from build123d import *

# Parameters (mm, degrees)
SKETCH1_W                      = 50.8
SKETCH1_H                      = 19.05
BOSS_EXTRUDE1_DEPTH            = 25.4
CUT_EXTRUDE1_DEPTH             = 38.162422217
CUT_EXTRUDE1_DEPTH_BACK        = 38.1
M4X0_7_TAPPED_HOLE1_D          = 3.3
M4X0_7_TAPPED_HOLE1_DEPTH      = 10.1092
M4X0_7_TAPPED_HOLE1_TIP        = 0.991420021
BOSS_EXTRUDE4_DEPTH            = 12.7
M2X0_4_TAPPED_HOLE1_AT_2_COUNT = 2
M2X0_4_TAPPED_HOLE1_AT_2_PITCH = 12.7
CUT_EXTRUDE2_DEPTH             = 12.7


with BuildPart() as part:
    # Sketch1 → Boss-Extrude1 (new body)
    with BuildSketch(Plane.XY):
        Rectangle(SKETCH1_W, SKETCH1_H)
    extrude(amount=BOSS_EXTRUDE1_DEPTH)

    # Sketch2 → Cut-Extrude1 (cut, two sides)
    with BuildSketch(Plane(origin=(0, 0, 0), x_dir=(-1, 0, 0), z_dir=(0, 0, -1))) as cut_extrude1_sk:
        Polygon((-6.461803399, -9.525), (-6.35, -9.525), (-12.7, 3.175), (12.7, 3.175), (6.35, -9.525), (6.461803399, -9.525), (12.861803399, 3.275), (-12.861803399, 3.275), align=None)
        Polygon((-12.7, 3.175), (-6.35, -9.525), (6.35, -9.525), (12.7, 3.175), align=None)
    extrude(amount=CUT_EXTRUDE1_DEPTH, mode=Mode.SUBTRACT)
    extrude(cut_extrude1_sk.sketch, amount=-CUT_EXTRUDE1_DEPTH_BACK, mode=Mode.SUBTRACT)

    # M4x0.7 Tapped Hole1
    with Locations(Plane(origin=(0, 9.525, 0), x_dir=(1, 0, 0), z_dir=(0, 1, 0))):
        with Locations((-19.05, -12.7), (19.05, -12.7)):
            Hole(M4X0_7_TAPPED_HOLE1_D / 2, depth=M4X0_7_TAPPED_HOLE1_DEPTH)
            with Locations((0, 0, -(M4X0_7_TAPPED_HOLE1_DEPTH + M4X0_7_TAPPED_HOLE1_TIP / 2))):  # 118° drill point
                Cone(0, M4X0_7_TAPPED_HOLE1_D / 2, M4X0_7_TAPPED_HOLE1_TIP, mode=Mode.SUBTRACT)

    # Sketch8 → Boss-Extrude4 (add)
    with BuildSketch(Plane.XZ.offset(9.525)):
        Polygon((25.4, 25.4), (63.5, -6.35), (63.5, -31.75), (25.4, 0), align=None)
    boss_extrude4 = extrude(amount=-BOSS_EXTRUDE4_DEPTH)

    # Sketch19 → M2x0.4 Tapped Hole1 (revolve, cut)
    with BuildSketch(Plane(origin=(63.5, -3.175, -22.225), x_dir=(0, 0, -1), z_dir=(0, 1, 0))):
        Polygon((0, 0), (0, 6.830688495), (0.8, 6.35), (0.8, 0), align=None)
    m2x0_4_tapped_hole1 = revolve(axis=Axis((69.85, -3.175, -22.225), (-1, 0, 0)), mode=Mode.SUBTRACT)

    # M2x0.4 Tapped Hole1 at 2: M2x0.4 Tapped Hole1 ×2
    with Locations(*[(0, 0, i * M2X0_4_TAPPED_HOLE1_AT_2_PITCH) for i in range(1, M2X0_4_TAPPED_HOLE1_AT_2_COUNT)]):
        add(m2x0_4_tapped_hole1, mode=Mode.SUBTRACT)

    # Sketch20 → Cut-Extrude2 (cut)
    with BuildSketch(Plane(origin=(0, 3.175, 0), x_dir=(1, 0, 0), z_dir=(0, 1, 0))):
        Polygon((57.404, 26.67), (63.5, 26.67), (63.5, 31.75), align=None)
    cut_extrude2 = extrude(amount=-CUT_EXTRUDE2_DEPTH, mode=Mode.SUBTRACT)

    # Mirror1: Boss-Extrude4, M2x0.4 Tapped Hole1, Cut-Extrude2 across plane
    add(boss_extrude4.mirror(Plane(origin=(0, 0, 0), x_dir=(0, 0, 1), z_dir=(1, 0, 0))))
    add(m2x0_4_tapped_hole1.mirror(Plane(origin=(0, 0, 0), x_dir=(0, 0, 1), z_dir=(1, 0, 0))), mode=Mode.SUBTRACT)
    add(cut_extrude2.mirror(Plane(origin=(0, 0, 0), x_dir=(0, 0, 1), z_dir=(1, 0, 0))), mode=Mode.SUBTRACT)

    # Mirror1 copy 1 sketch → Mirror1 copy 1 (revolve, cut)
    with BuildSketch(Plane(origin=(-63.5, -3.175, -9.525), x_dir=(0, 0, -1), z_dir=(0, 1, 0))):
        Polygon((0, 0), (0, -6.830688495), (0.8, -6.35), (0.8, 0), align=None)
    revolve(axis=Axis((-69.85, -3.175, -9.525), (-1, 0, 0)), mode=Mode.SUBTRACT)


solid = part.part
The model under review builds one solid part; all positions refer to its coordinate system, in mm. A direction names the side the tool comes from. Round coordinates to 2 decimals unless told otherwise and drop trailing zeros. Loops run counter-clockwise (first coordinate to the right, second up) from the corner with the lowest first, then second, coordinate; pieces in that order, holes last. Notation, with made-up numbers: M 74,32 L 104,32 A19 ccw 104,59 Z; hole C 33.25,-40 d2. An arc over 180 degrees is marked long. Answer as a JSON object with one key per item and string values.
Item 1: We need section C-C, the plane y = -8. State the section outline as (x, z) points, and give its area (3 significant figures).
Check sheet entries:
{"outline": "M -63.5,-26.67 L -57.4,-26.67 L -25.4,0 L -7.22,0 L -7.22,25.4 L -25.4,25.4 L -63.5,-6.35 Z; M 7.22,0 L 25.4,0 L 57.4,-26.67 L 63.5,-26.67 L 63.5,-6.35 L 25.4,25.4 L 7.22,25.4 Z", "area": "2,830 mm2"}
Item 2: Tool access review of faces 4 (the face through (41.6, -3.3, -13.5)), 5 (the face through (-17.834, 4.4, 11.585)), 6 (the face through (-45, 3.175, 0)): name each direction out of +Z, -Z, +X, -X, +Y, -Y from which nothing blocks a thin tool from reaching the whole face with its end or side.
Check sheet entries:
{"face 4": "-Z, +Y, -Y", "face 5": "+Y", "face 6": "+Z, -Z, -X, +Y"}
Item 3: We need section A-A, the plane z = -4.5. State the section outline as (x, y) points (3 decimals), and give its area (3 significant figures).
Check sheet entries:
{"outline": "M -61.28,-9.525 L -30.8,-9.525 L -30.8,3.175 L -61.28,3.175 Z; M 30.8,-9.525 L 61.28,-9.525 L 61.28,3.175 L 30.8,3.175 Z", "area": "774 mm2"}
Item 4: Clearance check with flat-ended pins moving along their axes: P1, Ø1, axis at x = -48.5, y = 0.5, coming from the +Z side; P2, Ø11.5, axis at x = -53.5, z = -8.5, coming from the +Y side (3 decimals); P3, Ø6, axis at x = -23, y = -5, coming from the -Z side; P4, Ø2, axis at y = 6, z = -21, coming from the -X side. State where each tip first meets the part, or that it passes through.
Check sheet entries:
{"P1": "z = 6.57", "P2": "y = 3.175", "P3": "z = -0.5", "P4": "through"}
Item 5: We need section D-D, the plane z = -14. State the section outline as (x, y) points (3 decimals), and give its area (3 significant figures).
Check sheet entries:
{"outline": "M -63.5,-9.525 L -42.2,-9.525 L -42.2,3.175 L -63.5,3.175 Z; M 42.2,-9.525 L 63.5,-9.525 L 63.5,3.175 L 42.2,3.175 Z", "area": "541 mm2"}
Item 6: We need section B-B, the plane y = 7.5. State the section outline as (x, z) points.
Check sheet entries:
{"outline": "M -25.4,0 L 25.4,0 L 25.4,25.4 L -25.4,25.4 Z; hole C -19.05,12.7 d3.3; hole C 19.05,12.7 d3.3"}
Item 7: For line 1 along Z through (x, y) = (19.05, 7); line 2 along X through (y, z) = (6.5, 17); line 3 along Y through (x, z) = (-10.5, 22.5) (3 decimals), list the stretches that pass through material, from the lowest coordinate up.
Check sheet entries:
{"line 1": "0 to 11.05, 14.35 to 25.4", "line 2": "-25.4 to 25.4", "line 3": "-9.525 to -1.449, 3.275 to 9.525"}
Item 8: The part is to be moulded in two halves that separate along Y. For faces 1 (the face through (9.707, -3.035, 12.522)), 2 (the face through (45, 3.175, 0)), 3 (the face through (-63.5, -3, -16)), say which applies: +Y half, -Y half, draft (parallel to the pull), parting line (faces both ways), or undercut.
Check sheet entries:
{"face 1": "undercut", "face 2": "+Y half", "face 3": "draft"}
